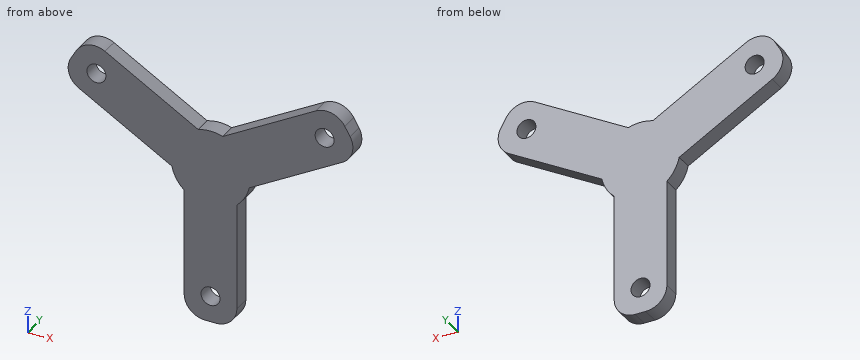
from build123d import *

# Parameters (mm, degrees)
SKETCH1_R           = 7.5
SKETCH1_R_2         = 5
SKETCH1_R_3         = 1.8
BOSS_EXTRUDE1_DEPTH = 3.175


with BuildPart() as part:
    # Sketch1 → Boss-Extrude1 (new body)
    with BuildSketch(Plane(origin=(0, 0, 0), x_dir=(1, 0, 0), z_dir=(0, 1, 0))):
        Circle(SKETCH1_R)
        Circle(SKETCH1_R_2, mode=Mode.SUBTRACT)
        with BuildLine():
            Line((2.5, 4.330127019), (-2.5, -4.330127019))
            Line((-2.5, -4.330127019), (20.016660498, -17.330127019))
            ThreePointArc((20.016660498, -17.330127019), (23.051936679, -17.729728709), (25.480762114, -15.866025404))
            Line((25.480762114, -15.866025404), (26.480762114, -14.133974596))
            ThreePointArc((26.480762114, -14.133974596), (26.880363804, -11.098698416), (25.016660498, -8.669872981))
            Line((25.016660498, -8.669872981), (2.5, 4.330127019))
        make_face()
        with Locations((21.650635095, -12.5)):
            Circle(SKETCH1_R_3, mode=Mode.SUBTRACT)
        with BuildLine():
            Line((-5, 0), (5, 0))
            Line((5, 0), (5, 26))
            ThreePointArc((5, 26), (3.828427125, 28.828427125), (1, 30))
            Line((1, 30), (-1, 30))
            ThreePointArc((-1, 30), (-3.828427125, 28.828427125), (-5, 26))
            Line((-5, 26), (-5, 0))
        make_face()
        with Locations((0, 25)):
            Circle(SKETCH1_R_3, mode=Mode.SUBTRACT)
        with BuildLine():
            Line((2.5, -4.330127019), (-2.5, 4.330127019))
            Line((-2.5, 4.330127019), (-25.016660498, -8.669872981))
            ThreePointArc((-25.016660498, -8.669872981), (-26.880363804, -11.098698416), (-26.480762114, -14.133974596))
            Line((-26.480762114, -14.133974596), (-25.480762114, -15.866025404))
            ThreePointArc((-25.480762114, -15.866025404), (-23.051936679, -17.729728709), (-20.016660498, -17.330127019))
            Line((-20.016660498, -17.330127019), (2.5, -4.330127019))
        make_face()
        with Locations((-21.650635095, -12.5)):
            Circle(SKETCH1_R_3, mode=Mode.SUBTRACT)
    extrude(amount=BOSS_EXTRUDE1_DEPTH)


solid = part.part
Read the model definition and answer for the solid it produces. Units are mm, in the model's axes. Round coordinates to 2 decimals unless told otherwise and drop trailing zeros. Loops run counter-clockwise (first coordinate to the right, second up) from the corner with the lowest first, then second, coordinate; pieces in that order, holes last.
Q1. This flat-tipped pin is pushed along its axis until it touches: pin 1 (3 mm diameter, centred on x = 0, z = -25, fed in from +Y). Where does it stop, or does it pass through?
Q2. Section A-A on x = 0 is taken. Write down the section's boundary in (y, z) (3 decimals), and give its area (3 significant figures).
Q3. Section D-D on z = -10 is taken. Write down the section's boundary in (x, y) (3 decimals), and give its area (4 significant figures).
Q4. Section B-B on z = 12.5 is taken. Write down the section's boundary in (x, y) (3 decimals), and give its area (3 significant figures).
Q5. Section C-C on y = 1.3 is taken. Write down the section's boundary in (x, z), and give its area (3 significant figures).
Q6. Consider probe 1 along X at (y, z) = (0.7, -25); probe 2 along X at (y, z) = (1.95, 12.5); probe 3 along Z at (x, y) = (0, 1.6). Determine where each line is inside the solid, lowest interval first.
Output:
1. pin 1: passes through
2. outline: (0, -30) - (3.175, -30) - (3.175, -26.8) - (0, -26.8) - close; (0, -23.2) - (3.175, -23.2) - (3.175, 7.5) - (0, 7.5) - close
2. area: 108 mm2
3. outline: (-5, 0) - (5, 0) - (5, 3.175) - (-5, 3.175) - close
3. area: 31.75 mm2
4. outline: (-27, 0) - (-23.451, 0) - (-23.451, 3.175) - (-27, 3.175) - close; (-19.851, 0) - (-11.651, 0) - (-11.651, 3.175) - (-19.851, 3.175) - close; (11.651, 0) - (19.851, 0) - (19.851, 3.175) - (11.651, 3.175) - close; (23.451, 0) - (27, 0) - (27, 3.175) - (23.451, 3.175) - close
4. area: 74.6 mm2
5. outline: (-26.48, 14.13) arc R4 ccw to (-25.02, 8.67) - (-7.34, -1.54) arc R7.5 ccw to (-5, -5.59) - (-5, -26) arc R4 ccw to (-1, -30) - (1, -30) arc R4 ccw to (5, -26) - (5, -5.59) arc R7.5 ccw to (7.34, -1.54) - (25.02, 8.67) arc R4 ccw to (26.48, 14.13) - (25.48, 15.87) arc R4 ccw to (20.02, 17.33) - (2.34, 7.13) arc R7.5 ccw to (-2.34, 7.13) - (-20.02, 17.33) arc R4 ccw to (-25.48, 15.87) - close; hole circle Ø3.6 at (-21.65, 12.5); hole circle Ø3.6 at (0, -25); hole circle Ø3.6 at (21.65, 12.5)
5. area: 819 mm2
6. probe 1: x = -5 to -1.8, 1.8 to 5
6. probe 2: x = -27 to -23.45, -19.85 to -11.65, 11.65 to 19.85, 23.45 to 27
6. probe 3: z = -30 to -26.8, -23.2 to 7.5
